Source: CAD feature listing. Evaluate the final solid. Frame: model axes, mm. A direction names the side the tool comes from. Coordinates: 2 decimals unless noted, no trailing zeros. Order: outer loops, then holes, each group sorted by start corner. A loop starts at its lowest first (then second) coordinate and runs counter-clockwise, first axis right, second up.
Item 1: Section B-B on z = -9. Return the cut outline in (x, y).
Item 2: Reachability of faces 4 (the flat face through (81, -10, 24.781)), 5 (the flat face through (-36.656, 53, 4)), 6 (the flat face through (-71, -10, -43.519)), 7 (the flat face through (-7, 0, 4)), 8 (the flat face through (23.944, 53, 4)) from +Z, -Z, +X, -X, +Y, -Y: full face, straight path, thin tool, end or side. Return the list, or none.
Item 3: Contact query for flat-ended pins moving along their axis: P1, Ø2.5, axis at x = -34.5, z = 7.5, coming from the +Y side; P2, Ø1.5, axis at x = 55, z = 36.5, coming from the +Y side; P3, Ø4, axis at y = 49, z = 32.5, coming from the +X side. Output: stop coordinate, or through.
Item 4: Section A-A on y = 6. Return the cut outline in (x, z).
Item 5: Section C-C on x = -82.5. Return the cut outline in (y, z), then the cut area to 3 significant figures.
Item 6: Ray query, line 1 (X direction, y = 56.5, z = -5.5); line 2 (Z direction, x = -18.5, y = 170.5); line 3 (X direction, y = 161, z = 33). Return the intervals inside material, ascending.
Item 7: Mould query, pull axis Z, two halves, no side actions, for faces 1 (the cylindrical face through (77.93, -7.6, 49.08)), 2 (the flat face through (-7, 90, 31.781)), 3 (the flat face through (-66.656, -10, 52)). Classes: released by +Z, released by -Z, zero draft, split by the parting line, or undercut.
Item 8: Section D-D on x = -50.5. Return the cut outline in (y, z).
from build123d import *

# Parameters (mm, degrees)
SKETCH_1_W          = 60.6
SKETCH_1_H          = 63.3
SKETCH_1_W_2        = 54.6
SKETCH_1_H_2        = 57.3
EXTRUDE_1_DEPTH     = 118
SKETCH_2_W          = 60.6
SKETCH_2_H          = 3
EXTRUDE_2_DEPTH     = 65
CUT_EXTRUDE_1_DEPTH = 65
SKETCH_4_W          = 180.6
SKETCH_4_H          = 103.3
EXTRUDE_3_DEPTH     = 5
CUT_EXTRUDE_2_DEPTH = 5
EXTRUDE_START       = 10
EXTRUDE_4_DEPTH     = 10
SKETCH_8_R          = 0.75
CUT_EXTRUDE_3_DEPTH = 10
SKETCH_9_R          = 1.5
CUT_EXTRUDE_4_DEPTH = 10


with BuildPart() as part:
    # 草图1 → 凸台-拉伸1 (new body)
    with BuildSketch(Plane(origin=(0, 0, 0), x_dir=(1, 0, 0), z_dir=(0, 1, 0))):
        with Locations((-6.35625, -3.13125)):
            Rectangle(SKETCH_1_W, SKETCH_1_H)
        with Locations((-6.35625, -3.13125)):
            Rectangle(SKETCH_1_W_2, SKETCH_1_H_2, mode=Mode.SUBTRACT)
    extrude(amount=EXTRUDE_1_DEPTH)

    # 草图2 → 凸台-拉伸2 (add)
    with BuildSketch(Plane(origin=(0, 118, 0), x_dir=(1, 0, 0), z_dir=(0, 1, 0))):
        with Locations((-6.35625, 27.01875)):
            Rectangle(SKETCH_2_W, SKETCH_2_H)
        with Locations((-6.35625, -33.28125)):
            Rectangle(SKETCH_2_W, SKETCH_2_H)
    extrude(amount=EXTRUDE_2_DEPTH)

    # 草图3 → 切除-拉伸1 (cut)
    with BuildSketch(Plane(origin=(0, 0, -28.51875), x_dir=(-1, 0, 0), z_dir=(0, 0, -1))):
        with BuildLine():
            Line((36.65625, 183), (6.356250104, 183))
            ThreePointArc((6.356250104, 183), (19.282049563, 178.802351128), (27.275306551, 167.811246068))
            Line((27.275306551, 167.811246068), (36.65625, 139))
            Line((36.65625, 139), (36.65625, 183))
        make_face()
        with BuildLine():
            Line((-23.94375, 183), (-23.94375, 139))
            Line((-23.94375, 139), (-14.562806551, 167.811246068))
            ThreePointArc((-14.562806551, 167.811246068), (-6.569549479, 178.802351188), (6.356250104, 183))
            Line((6.356250104, 183), (-23.94375, 183))
        make_face()
    extrude(amount=-CUT_EXTRUDE_1_DEPTH, mode=Mode.SUBTRACT)

    # 草图4 → 凸台-拉伸3 (add)
    with BuildSketch(Plane.XZ):
        with Locations((-6.35625, 3.13125)):
            Rectangle(SKETCH_4_W, SKETCH_4_H)
    extrude(amount=EXTRUDE_3_DEPTH)

    # 草图5 → 切除-拉伸2 (cut)
    with BuildSketch(Plane.XZ.offset(5)):
        with BuildLine():
            ThreePointArc((-76.65625, -48.51875), (-90.798385624, -42.660885624), (-96.65625, -28.51875))
            Line((-96.65625, -28.51875), (-96.65625, -48.51875))
            Line((-96.65625, -48.51875), (-76.65625, -48.51875))
        make_face()
        with BuildLine():
            Line((-76.65625, 54.78125), (-86.65625, 54.78125))
            Line((-86.65625, 54.78125), (-96.65625, 54.78125))
            Line((-96.65625, 54.78125), (-96.65625, 34.78125))
            ThreePointArc((-96.65625, 34.78125), (-90.798385624, 48.923385624), (-76.65625, 54.78125))
        make_face()
        with BuildLine():
            Line((83.94375, 54.78125), (63.94375, 54.78125))
            ThreePointArc((63.94375, 54.78125), (78.085885624, 48.923385624), (83.94375, 34.78125))
            Line((83.94375, 34.78125), (83.94375, 54.78125))
        make_face()
        with BuildLine():
            Line((83.94375, -48.51875), (83.94375, -28.51875))
            ThreePointArc((83.94375, -28.51875), (78.085885624, -42.660885624), (63.94375, -48.51875))
            Line((63.94375, -48.51875), (83.94375, -48.51875))
        make_face()
    extrude(amount=-CUT_EXTRUDE_2_DEPTH, mode=Mode.SUBTRACT)

    # 草图6 → 凸台-拉伸4 (add)
    with BuildSketch(Plane.XZ.offset(5).offset(EXTRUDE_START)):
        with BuildLine():
            Line((-76.317762068, 49.78125), (-66.65625, 49.78125))
            Line((-66.65625, 49.78125), (-66.65625, 54.78125))
            Line((-66.65625, 54.78125), (-76.65625, 54.78125))
            ThreePointArc((-76.65625, 54.78125), (-90.798385624, 48.923385624), (-96.65625, 34.78125))
            Line((-96.65625, 34.78125), (-96.65625, 24.78125))
            Line((-96.65625, 24.78125), (-91.65625, 24.78125))
            Line((-91.65625, 24.78125), (-91.65625, 34.442762068))
            ThreePointArc((-91.65625, 34.442762068), (-87.265551911, 45.390551911), (-76.317762068, 49.78125))
        make_face()
        with BuildLine():
            Line((78.94375, 24.78125), (83.94375, 24.78125))
            Line((83.94375, 24.78125), (83.94375, 34.78125))
            ThreePointArc((83.94375, 34.78125), (78.085885624, 48.923385624), (63.94375, 54.78125))
            Line((63.94375, 54.78125), (53.94375, 54.78125))
            Line((53.94375, 54.78125), (53.94375, 49.78125))
            Line((53.94375, 49.78125), (63.605262068, 49.78125))
            ThreePointArc((63.605262068, 49.78125), (74.553051911, 45.390551911), (78.94375, 34.442762068))
            Line((78.94375, 34.442762068), (78.94375, 24.78125))
        make_face()
        with BuildLine():
            Line((78.94375, -28.180262068), (78.94375, -18.51875))
            Line((78.94375, -18.51875), (83.94375, -18.51875))
            Line((83.94375, -18.51875), (83.94375, -28.51875))
            ThreePointArc((83.94375, -28.51875), (78.085885624, -42.660885624), (63.94375, -48.51875))
            Line((63.94375, -48.51875), (53.94375, -48.51875))
            Line((53.94375, -48.51875), (53.94375, -43.51875))
            Line((53.94375, -43.51875), (63.605262068, -43.51875))
            ThreePointArc((63.605262068, -43.51875), (74.553051911, -39.128051911), (78.94375, -28.180262068))
        make_face()
        with BuildLine():
            Line((-91.65625, -18.51875), (-96.65625, -18.51875))
            Line((-96.65625, -18.51875), (-96.65625, -28.51875))
            ThreePointArc((-96.65625, -28.51875), (-90.798385624, -42.660885624), (-76.65625, -48.51875))
            Line((-76.65625, -48.51875), (-66.65625, -48.51875))
            Line((-66.65625, -48.51875), (-66.65625, -43.51875))
            Line((-66.65625, -43.51875), (-76.317762068, -43.51875))
            ThreePointArc((-76.317762068, -43.51875), (-87.265551911, -39.128051911), (-91.65625, -28.180262068))
            Line((-91.65625, -28.180262068), (-91.65625, -18.51875))
        make_face()
    extrude(amount=-EXTRUDE_4_DEPTH)

    # 草图8 → 切除-拉伸3 (cut)
    with BuildSketch(Plane.XY.offset(34.78125)):
        with Locations((-6.35625, 177.5)):
            Circle(SKETCH_8_R)
        with Locations((10.14375, 161)):
            Circle(SKETCH_8_R)
        with Locations((-6.35625, 144.5)):
            Circle(SKETCH_8_R)
        with Locations((-22.85625, 161)):
            Circle(SKETCH_8_R)
    extrude(amount=-CUT_EXTRUDE_3_DEPTH, mode=Mode.SUBTRACT)

    # 草图9 → 切除-拉伸4 (cut)
    with BuildSketch(Plane(origin=(0, 0, -28.51875), x_dir=(-1, 0, 0), z_dir=(0, 0, -1))):
        with Locations((6.35625, 161)):
            Circle(SKETCH_9_R)
    extrude(amount=-CUT_EXTRUDE_4_DEPTH, mode=Mode.SUBTRACT)


solid = part.part
Answer list:
1. outline: (-96.66, -5) - (83.94, -5) - (83.94, 0) - (23.94, 0) - (23.94, 118) - (20.94, 118) - (20.94, 0) - (-33.66, 0) - (-33.66, 118) - (-36.66, 118) - (-36.66, 0) - (-96.66, 0) - close
2. face 4: +X, -X, -Y
2. face 5: +Z, -Z, -X, +Y
2. face 6: -Y
2. face 7: +Y
2. face 8: +Z, -Z, +X, +Y
3. P1: stops at y = 118
3. P2: stops at y = 0
3. P3: stops at x = 23.94
4. outline: (-36.66, -28.52) - (23.94, -28.52) - (23.94, 34.78) - (-36.66, 34.78) - close; hole (-33.66, -25.52) - (20.94, -25.52) - (20.94, 31.78) - (-33.66, 31.78) - close
5. outline: (-15, -47.65) - (0, -47.65) - (0, 53.91) - (-15, 53.91) - (-15, 48.6) - (-5, 48.6) - (-5, -42.34) - (-15, -42.34) - close
5. area: 614 mm2
6. line 1: x = -36.66 to -33.66, 20.94 to 23.94
6. line 2: z = -28.52 to -25.52, 31.78 to 34.78
6. line 3: x = -29.49 to -23.61, -22.11 to 9.39, 10.89 to 16.78
7. face 1: released by +Z
7. face 2: undercut
7. face 3: zero draft
8. outline: (-5, -48.52) - (0, -48.52) - (0, 54.78) - (-5, 54.78) - close
